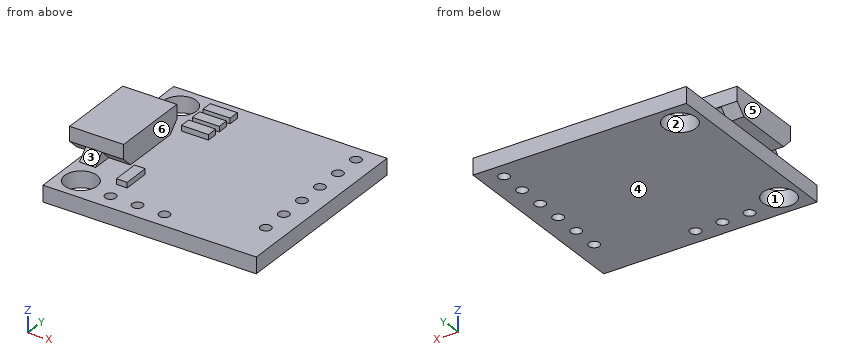
from build123d import *

# Parameters (mm, degrees)
SKETCH1_W           = 20.066
SKETCH1_H           = 18.415
SKETCH1_R           = 1.524
EXTRUDE1_DEPTH      = 1.524
EXTRUDE2_DEPTH      = 1.143
EXTRUDE2_DEPTH_BACK = 3.937
SKETCH3_R           = 0.508
EXTRUDE3_DEPTH      = 15.663683105
LPATTERN1_COUNT     = 6
LPATTERN1_PITCH     = 2.54
SKETCH4_R           = 0.508
EXTRUDE4_DEPTH      = 15.663683105
LPATTERN2_COUNT     = 3
LPATTERN2_PITCH     = 2.54
SKETCH5_W           = 2.54
SKETCH5_H           = 1.016
SKETCH5_W_2         = 1.016
SKETCH5_H_2         = 2.54
KEEPAWAY_DEPTH      = 0.508
EXTRUDE6_START      = -1.524
EXTRUDE6_DEPTH      = 1.524


with BuildPart() as part:
    # Sketch1 → Extrude1 (new body)
    with BuildSketch(Plane.XY):
        Rectangle(SKETCH1_W, SKETCH1_H)
        with Locations(Location((-7.9502, 6.985, 0), (0, 0, 180))):
            Circle(SKETCH1_R, mode=Mode.SUBTRACT)
        with Locations(Location((-7.9502, -6.985, 0), (0, 0, 180))):
            Circle(SKETCH1_R, mode=Mode.SUBTRACT)
    extrude(amount=EXTRUDE1_DEPTH)

    # Sketch2 → Extrude2 (add, two sides: drawn at the far end of the back side and taken through both)
    with BuildSketch(Plane.ZY.offset(10.033).offset(-EXTRUDE2_DEPTH_BACK)):
        Polygon((3.8354, 3.7465), (3.8354, -3.7465), (2.481413228, -3.7465), (1.524, -2.789086772), (1.524, 2.789086772), (2.481413228, 3.7465), align=None)
    extrude(amount=EXTRUDE2_DEPTH + EXTRUDE2_DEPTH_BACK)

    # Sketch3 → Extrude3 (cut, through all)
    with BuildSketch(Plane.XY.offset(1.524)):
        with Locations((8.128, 7.6835)):
            Circle(SKETCH3_R)
    extrude3 = extrude(amount=-EXTRUDE3_DEPTH, mode=Mode.SUBTRACT)

    # LPattern1: Extrude3 ×6
    with Locations(*[(0, -i * LPATTERN1_PITCH, 0) for i in range(1, LPATTERN1_COUNT)]):
        add(extrude3, mode=Mode.SUBTRACT)

    # Sketch4 → Extrude4 (cut, through all)
    with BuildSketch(Plane.XY.offset(1.524)):
        with Locations((-4.699, -7.6835)):
            Circle(SKETCH4_R)
    extrude4 = extrude(amount=-EXTRUDE4_DEPTH, mode=Mode.SUBTRACT)

    # LPattern2: Extrude4 ×3
    with Locations(*[(i * LPATTERN2_PITCH, 0, 0) for i in range(1, LPATTERN2_COUNT)]):
        add(extrude4, mode=Mode.SUBTRACT)

    # Sketch5 → KeepAway (add)
    with BuildSketch(Plane.XY.offset(1.524)):
        with Locations((-4.4196, 7.3533)):
            Rectangle(SKETCH5_W, SKETCH5_H)
        with Locations((-4.4196, 5.8293)):
            Rectangle(SKETCH5_W, SKETCH5_H)
        with Locations((-4.4196, 4.3053)):
            Rectangle(SKETCH5_W, SKETCH5_H)
        with Locations((-4.826, -4.6355)):
            Rectangle(SKETCH5_W_2, SKETCH5_H_2)
    extrude(amount=KEEPAWAY_DEPTH)

    # Sketch6 → Extrude6 (add)
    with BuildSketch(Plane.ZY.offset(11.176).offset(EXTRUDE6_START)):
        Polygon((1.524, 4.6355), (1.524, 2.789086772), (2.481413228, 3.7465), align=None)
        Polygon((1.524, -2.789086772), (1.524, -4.6355), (2.481413228, -3.7465), align=None)
    extrude(amount=-EXTRUDE6_DEPTH)


solid = part.part
Input: part model. Units: mm. Frame: model coordinates. Face numbers are marked on the shaded views. A direction names the side the tool comes from. Coordinates: 2 decimals unless noted, no trailing zeros. Loops run counter-clockwise (first coordinate to the right, second up) from the corner with the lowest first, then second, coordinate; pieces in that order, holes last. Notation, with made-up numbers: (22.25, -25.5) -> (48.25, -25.5) arc R3 ccw to (48.25, -21.5) -> close; hole circle Ø5 at (3, 5.5). An arc over 180 degrees is marked (long way). One line per item, written item: value.
(1) Pin query (flat end, axial travel): pin 1 Ø0.8 at (x, y) = (-5, 5.5) entering from +Z; pin 2 Ø1.5 at (y, z) = (2.5, 2.5) entering from +X; pin 3 Ø1.5 at (x, z) = (-9, 3.5) entering from -Y; pin 4 Ø5 at (x, y) = (-7.95, 6.98) entering from -Z. Return the tip coordinate at first contact, or that it passes through.
Answer below:
pin 1: stops at z = 2.03
pin 2: stops at x = -6.1
pin 3: stops at y = -3.75
pin 4: stops at z = 0
(2) Cut plane D-D (y = -6.75). Output: boundary loops of the cut face in (x, z), then the cut area to 3 significant figures.
Answer below:
outline: (-10.03, 0) -> (-9.46, 0) -> (-9.46, 1.52) -> (-10.03, 1.52) -> close; (-6.44, 0) -> (10.03, 0) -> (10.03, 1.52) -> (-6.44, 1.52) -> close
area: 26.0 mm2
(3) Cut plane C-C (x = 4.5). Output: boundary loops of the cut face in (y, z).
Answer below:
outline: (-9.21, 0) -> (9.21, 0) -> (9.21, 1.52) -> (-9.21, 1.52) -> close
(4) Draft query along Y for the marked faces 1, 2, 3 and 4. Return one class per face: pulls with the +Y half, pulls with the -Y half, needs draft (parallel to the pull), parting line crosses it, or undercut.
Answer below:
face 1: undercut
face 2: undercut
face 3: pulls with the -Y half
face 4: needs draft
(5) Set-up query: the marked faces 5 and 6. Return all of +Z, -Z, +X, -X, +Y, -Y with unobstructed straight access to the full face (end or side cutting, diameter ignored); none if empty.
Answer below:
face 5: +Z, -Z, -X, +Y, -Y
face 6: +Z, +X, +Y, -Y
(6) Ray query, line 1 along Y through (x, z) = (-9, 1.1); line 2 along X through (y, z) = (4, 1.7); line 3 along Z through (x, y) = (-5.5, -7.25). Return the intervals inside material, ascending.
Answer below:
line 1: y = -9.21 to -8.09, -5.88 to 5.88, 8.09 to 9.21
line 2: x = -9.65 to -8.13, -5.69 to -3.15
line 3: z = 0 to 1.52
(7) Cut plane A-A (z = 0.65). Give the number of separate pieces and of enclosed holes in the cut face, then the cut area to 3 significant figures.
Answer below:
separate pieces: 1
enclosed holes: 11
area: 348 mm2
(8) Cut plane B-B (y = 6). Output: boundary loops of the cut face in (x, z).
Answer below:
outline: (-10.03, 0) -> (-9.11, 0) -> (-9.11, 1.52) -> (-10.03, 1.52) -> close; (-6.79, 0) -> (10.03, 0) -> (10.03, 1.52) -> (-3.15, 1.52) -> (-3.15, 2.03) -> (-5.69, 2.03) -> (-5.69, 1.52) -> (-6.79, 1.52) -> close
